Design review of the part built by this model. Coordinates are the model's own, in mm. Round coordinates to 2 decimals unless told otherwise and drop trailing zeros. Write each loop counter-clockwise with the first axis right and the second up, starting at its lowest first coordinate (ties: lowest second). Pieces come first, ordered by that corner, then holes. Notation, with made-up numbers: (-32, -17) -> (4, -17) arc R16 ccw to (4, 13) -> close; hole circle Ø7 at (-1, 2.5). An arc over 180 degrees is marked (long way). One line per question, with ' | ' between items. Start each with the question number.
1) Insertion check: pin 1 Ø8 at (x, y) = (-59, -26.5) entering from +Z; pin 2 Ø2.5 at (x, y) = (32, 15) entering from +Z. Each pin has a flat end and moves straight along its axis. Give the tip position at first contact, or say it passes through.
2) Consider section D-D (z = 0.6). Count the separate pieces of the cut face and the enclosed holes in it, then the cut area to 3 significant figures.
3) Consider section A-A (y = 15). Give the boundary of the cut face in (x, z), then the cut area to 3 significant figures.
4) For probe 1 along Y at (x, z) = (32, 1.1); probe 2 along Y at (x, z) = (59, 1.3); probe 3 along X at (y, z) = (-14, 1.7), list the stretches that pass through material, from the lowest coordinate up.
5) Consider section B-B (x = -32). Give the boundary of the cut face in (y, z), then the cut area to 3 significant figures.
6) Mouldability with a two-part tool opening along X and no side actions: class faces 1 (the flat face through (-1, 8, 3)), 2 (the cylindrical face through (-33.2, 15.9, 1.5)), 3 (the cylindrical face through (-63.5, -31.07, 1.48)) as +X half, -X half, draft (parallel to the pull), parting line (faces both ways), or undercut.
7) Consider section C-C (y = 0). Give the boundary of the cut face in (x, z).
Autodesk Fusion 360 part; units mm, degrees
sketch "Sketch1" plane through (0, 0, 0) normal (0, 0, 1) x (1, 0, 0)
  line L0 (-60, 32.5) -> (0, 32.5)
  line L1 (0, -32.5) -> (-60, -32.5)
  line L2 (-65, -27.5) -> (-65, 27.5)
  arc A0 (-60, 32.5) -> (-65, 27.5) centre (-60, 27.5) ccw
  arc A1 (-65, -27.5) -> (-60, -32.5) centre (-60, -27.5) ccw
  circle A2 centre (-59, 26.5) radius 2.5
  circle A3 centre (-59, -26.5) radius 2.5
  circle A4 centre (0, 0) radius 3.5
  circle A5 centre (-56, 15) radius 1.5
  circle A6 centre (-56, -15) radius 1.5
  circle A7 centre (-32, 15) radius 1.5
  circle A8 centre (-32, -15) radius 1.5
  line L3 (0, 32.5) -> (0, -32.5) construction
  line L4 (65, -27.5) -> (65, 27.5)
  circle A9 centre (59, 26.5) radius 2.5
  arc A10 (60, -32.5) -> (65, -27.5) centre (60, -27.5) ccw
  circle A11 centre (32, 15) radius 1.5
  circle A12 centre (56, 15) radius 1.5
  circle A13 centre (56, -15) radius 1.5
  circle A14 centre (59, -26.5) radius 2.5
  arc A15 (65, 27.5) -> (60, 32.5) centre (60, 27.5) ccw
  line L5 (0, -32.5) -> (60, -32.5)
  line L6 (60, 32.5) -> (0, 32.5)
  circle A16 centre (32, -15) radius 1.5
  circle A17 centre (-18.75, 18.75) radius 1.5
  circle A18 centre (-18.75, -18.75) radius 1.5
  circle A19 centre (18.75, -18.75) radius 1.5
  circle A20 centre (18.75, 18.75) radius 1.5
  dimension "d1" = 65
  dimension "d3" = 32.5
  dimension "d4" = 32.5
  dimension "d5" = 5
  dimension "d6" = 5
  dimension "d9" = 5
  dimension "d10" = 6
  dimension "d11" = 6
  dimension "d12" = 5
  dimension "d13" = 6
  dimension "d14" = 6
  dimension "d21" = 7
  dimension "d24" = 9
  dimension "d25" = 9
  dimension "d26" = 30
  dimension "d27" = 3
  dimension "d28" = 3
  dimension "d29" = 17.5
  dimension "d30" = 3
  dimension "d31" = 3
  dimension "d32" = 30
  dimension "d33" = 17.5
  dimension "d34" = 24
  dimension "d35" = 65
  dimension "d36" = 65
  dimension "d41" = 3
  dimension "d42" = 3
  dimension "d43" = 37.5
  dimension "d44" = 13.75
  dimension "d45" = 18.75
extrude "Extrude4" add sketch "Sketch1" along normal blind 3
equation "d3 = ( 65 / 2 ) * 1 mm"
equation "d4 = d3"
equation "d6 = d5"
equation "d11 = d10"
equation "d12 = d9"
equation "d13 = d10"
equation "d14 = d10"
equation "d25 = d24"
equation "d28 = d27"
equation "d30 = d27"
equation "d31 = d27"
equation "d32 = d26"
equation "d33 = d29"
equation "d35 = d1"
equation "d36 = d1"
equation "d42 = d41"
equation "d44 = d3 - d43 / 2"
equation "d45 = ( 37.5 / 2 ) * 1 mm"
From the geometry:
1) pin 1: stops at z = 3 | pin 2: passes through
2) separate pieces: 1 | enclosed holes: 17 | area: 8,230 mm2
3) outline: (-65, 0) -> (-57.5, 0) -> (-57.5, 3) -> (-65, 3) -> close; (-54.5, 0) -> (-33.5, 0) -> (-33.5, 3) -> (-54.5, 3) -> close; (-30.5, 0) -> (30.5, 0) -> (30.5, 3) -> (-30.5, 3) -> close; (33.5, 0) -> (54.5, 0) -> (54.5, 3) -> (33.5, 3) -> close; (57.5, 0) -> (65, 0) -> (65, 3) -> (57.5, 3) -> close | area: 354 mm2
4) probe 1: y = -32.5 to -16.5, -13.5 to 13.5, 16.5 to 32.5 | probe 2: y = -32.5 to -29, -24 to 24, 29 to 32.5 | probe 3: x = -65 to -57.12, -54.88 to -33.12, -30.88 to 30.88, 33.12 to 54.88, 57.12 to 65
5) outline: (-32.5, 0) -> (-16.5, 0) -> (-16.5, 3) -> (-32.5, 3) -> close; (-13.5, 0) -> (13.5, 0) -> (13.5, 3) -> (-13.5, 3) -> close; (16.5, 0) -> (32.5, 0) -> (32.5, 3) -> (16.5, 3) -> close | area: 177 mm2
6) face 1: draft | face 2: undercut | face 3: -X half
7) outline: (-65, 0) -> (-3.5, 0) -> (-3.5, 3) -> (-65, 3) -> close; (3.5, 0) -> (65, 0) -> (65, 3) -> (3.5, 3) -> close
